Can you work these out from the model? Positions are in its coordinate system, mm. Face numbers are marked on the shaded views. A direction names the side the tool comes from. Give positions to 0.01 mm unless a question says otherwise; leave off trailing zeros. Loops run counter-clockwise (first coordinate to the right, second up) from the corner with the lowest first, then second, coordinate; pieces in that order, holes last. Notation, with made-up numbers: (-19, -39) - (6, -39) arc R17 cw to (6, -12) - close; hole circle Ø1 at (65, 77). An arc over 180 degrees is marked (long way). Answer as a JSON object with one key per item and string values. Group by question number.
Item 1: Suppose I cut it at B-B on y = 75.5. Write out the boundary of the cut face in (x, z).
Item 2: Thinking about a two-plate mould opening in Y: for the marked faces 1 and 2, which applies, pulls with the +Y half, pulls with the -Y half, needs draft (parallel to the pull), parting line crosses it, or undercut?
Item 3: Will these pins go through, and if not, where does the flat tip stop? pin 1 (2 mm diameter, centred on x = -1.5, y = 77, fed in from -Z); pin 2 (1 mm diameter, centred on y = 14.5, z = -2, fed in from -X); pin 3 (1 mm diameter, centred on y = 29.5, z = 2, fed in from -X).
Item 4: Suppose I cut it at A-A on z = 1.5. Write out the boundary of the cut face in (x, y), and give its area (3 significant figures).
Item 5: Which directions (+Z, -Z, +X, -X, +Y, -Y) give clear straight access to the entire face, cutting with the end or side of a thin tool? Please do the marked faces 3, 4 and 5.
Item 6: Please list where these lines run through material, in increasing order: L1, parallel to Y at x = 2.25, z = -2.5; L2, parallel to Y at x = -0.5, z = -1.25; L3, parallel to Z at x = 2, y = 65.
Autodesk Fusion 360 part; units mm, degrees
sketch "wedge side" plane through (0, 0, 0) normal (0, 1, 0) x (1, 0, 0)
  line L0 (0, 0) -> (5.0614, 5.0614)
  line L1 (0, 0) -> (7.1578, 0) construction
  line L2 (0, 0) -> (-1.312, -1.312)
  line L3 (-1.312, -1.312) -> (-10.924, -10.924)
  line L4 (12.4749, 3) -> (-4.8473, 3)
  line L5 (8.9736, -3) -> (-11.747, -3)
  line L6 (6, 3) -> (6, -3)
  dimension "d3" = 45
  dimension "d4" = 3
  dimension "d5" = 3
  dimension "d6" = 6
extrude "Extrude1" add sketch "wedge side" along normal blind 33 makes body 1
sketch "clip corners" plane through (0, 0, 3) normal (0, 0, 1) x (1, 0, 0)
  line L0 (-3, 0) -> (6, 0)
  line L1 (6, 0) -> (6, 33)
  line L2 (6, 33) -> (-3, 33)
  line L3 (-3, 33) -> (-3, 0)
  line L4 (-3, 31) -> (0, 33)
  line L5 (6, 16.5) -> (-3, 16.5) construction
  line L6 (-3, 2) -> (0, 0)
  dimension "d9" = 2
  dimension "d10" = 3
extrude "Extrude2" cut sketch "clip corners" against normal blind 10 contours L0 L3 L6 | L2 L3 L4 bodies 1
copy_body "CopyPasteBodies1" bodies 1 makes body 2
move_body "Move1" bodies 2 to x (1, 0, 0) y (0, -1, 0) z (0, 0, -1) at (0, 0, 0)
combine "Combine1" operation add target body 1 tool bodies 2
pattern_linear "R-Pattern1" count 3 spacing 66 along (0, 1, 0) both ways of bodies 1 makes body 3 at (6, -77, -1) makes body 4 at (6, 55, -1)
combine "Combine2" operation add target body 1 tool bodies 3 4
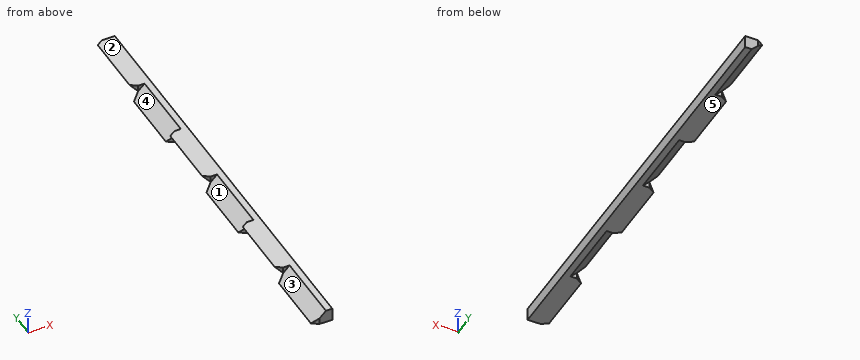
Worked out:
{
 "1": {"outline": "(-3, 3) - (3, -3) - (6, -3) - (6, 3) - close"},
 "2": {"face 1": "undercut", "face 2": "needs draft"},
 "3": {"pin 1": "stops at z = 0.5", "pin 2": "stops at x = 1.5", "pin 3": "stops at x = -2.5"},
 "4": {"outline": "(-1.5, -65) - (0, -66) - (1.5, -66) - (1.5, -99) - (6, -99) - (6, 99) - (0, 99) - (-1.5, 98) - (-1.5, 67) - (0, 66) - (1.5, 66) - (1.5, 33) - (0, 33) - (-1.5, 32) - (-1.5, 1) - (0, 0) - (1.5, 0) - (1.5, -33) - (0, -33) - (-1.5, -34) - close", "area": "1,180 mm2"},
 "5": {"face 3": "+Z, -X, -Y", "face 4": "+Z, -X", "face 5": "-Z, +X, -X, +Y, -Y"},
 "6": {"L1": "y = -99 to -66, -33 to 0, 33 to 66", "L2": "y = -98.67 to -66.33, -32.67 to -0.33, 33.33 to 65.67", "L3": "z = -3 to 2"}
}
